Source: three-view drawing plus pictorial views. Frame: mm from the lowest corner of the part. A direction names the side the tool comes from. Give positions to 0.01 mm unless a question says otherwise; leave off trailing zeros. Order: outer loops, then holes, each group sorted by start corner. A loop starts at its lowest first (then second) coordinate and runs counter-clockwise, first axis right, second up. Notation, with made-up numbers: M 23.25,-11 L 57.25,-11 A14 cw 57.25,1 Z; hole C -8.5,49 d11. An arc over 180 degrees is marked long. Use CSV: the item, a comma, the result in double quotes. Start each with the question number.
Item 1: Section query B-B on z = 20. Return loops of the section in (x, y).
Item 2: Section query D-D on y = 27. Return loops of the section in (x, z).
Item 3: Pull-direction query (X, two-part tool) for the marked faces 6, 7 and 8; classes: +X half, -X half, draft (parallel to the pull), parting line (faces both ways), or undercut.
Item 4: First-contact query: pin 1 (1 mm diameter, centred on x = 21.5, z = 11, fed in from -Y); pin 2 (12 mm diameter, centred on x = 33, y = 72.5, fed in from +Z); pin 3 (14 mm diameter, centred on y = 73.5, z = 6.5, fed in from -X). Flat tips, straight axial feed; report the tip coordinate or a pass-through.
Item 5: Section query A-A on y = 55. Return loops of the section in (x, z).
Item 6: Section query C-C on x = 40.75. Return loops of the section in (y, z), and give its area (3 significant figures).
Item 7: Ray query, probe 1 along X at (y, z) = (18.5, 20); probe 2 along Y at (x, z) = (35, 6); probe 3 along X at (y, z) = (45.5, 10.5). Return the intervals inside material, ascending. Write a range as from..to.
Item 8: Access query for the marked faces 1, 2, 3, 4 and 5. Directions: +Z, -Z, +X, -X, +Y, -Y. A direction counts if a zero-diameter tool reaches every point of the face in a straight line with its end or side. Return the directions, or none.
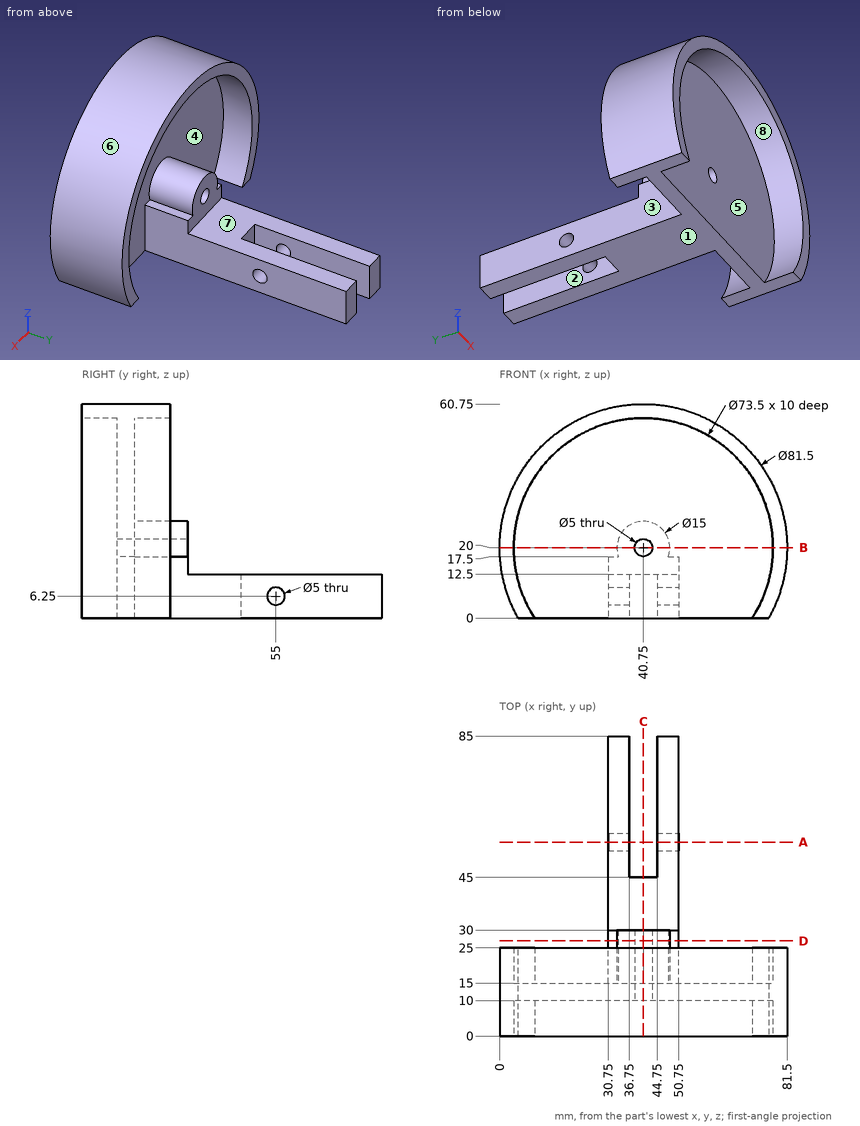
Verdict:
1,outline,"M 0,0 L 4,0 L 4,10 L 38.25,10 L 38.25,30 L 33.25,30 L 33.25,15 L 4,15 L 4,25 L 0,25 Z; M 43.25,10 L 77.5,10 L 77.5,0 L 81.5,0 L 81.5,25 L 77.5,25 L 77.5,15 L 48.25,15 L 48.25,30 L 43.25,30 Z"
2,outline,"M 30.75,0 L 50.75,0 L 50.75,17.5 L 47.82,17.5 A7.5 ccw long 33.68,17.5 L 30.75,17.5 Z; hole C 40.75,20 d5"
3,face 6,"parting line"
3,face 7,"draft"
3,face 8,"undercut"
4,pin 1,"y = 10"
4,pin 2,"z = 12.5"
4,pin 3,"x = 30.75"
5,outline,"M 30.75,0 L 36.75,0 L 36.75,3.75 L 30.75,3.75 Z; M 30.75,8.75 L 36.75,8.75 L 36.75,12.5 L 30.75,12.5 Z; M 44.75,0 L 50.75,0 L 50.75,3.75 L 44.75,3.75 Z; M 44.75,8.75 L 50.75,8.75 L 50.75,12.5 L 44.75,12.5 Z"
6,outline,"M 0,56.75 L 10,56.75 L 10,22.5 L 30,22.5 L 30,27.5 L 15,27.5 L 15,56.75 L 25,56.75 L 25,60.75 L 0,60.75 Z; M 10,0 L 45,0 L 45,12.5 L 30,12.5 L 30,17.5 L 10,17.5 Z"
6,area,"884 mm2"
7,probe 1,"0..4, 33.25..38.25, 43.25..48.25, 77.5..81.5"
7,probe 2,"10..52.51, 57.49..85"
7,probe 3,"30.75..36.75, 44.75..50.75"
8,face 1,"-Z, +X, -X, +Y, -Y"
8,face 2,"+Z, -Z, +Y"
8,face 3,"-Z, +Y"
8,face 4,"+Y"
8,face 5,"-Y"
